Here's the drawing with two shaded views (mm, measured from the low corner). I have some questions. Coordinates: 2 decimals unless noted, no trailing zeros. Order: outer loops, then holes, each group sorted by start corner. A loop starts at its lowest first (then second) coordinate and runs counter-clockwise, first axis right, second up. Notation, with made-up numbers: (-22.75, -9.5) -> (-8.75, -9.5) arc R36 ccw to (-8.75, 29.5) -> close; hole circle Ø7 at (46.25, -32). An arc over 180 degrees is marked (long way). Answer as a JSON object with one key per item and string values. Group by question number.
(1) I want a section at A-A, the plane z = 2.1. List the corners of the cut face in (x, y) for me.
(2) I want a section at B-B, the plane y = 5.5. List the corners of the cut face in (x, z) for me, plus the area to 3 significant figures.
(3) I need wall thicknesses on line 1 (X direction, y = 2, z = 1.25); line 2 (Y direction, x = 4.3, z = 2.3); line 3 (Y direction, x = 14.5, z = 0.65). Which ranges of each line are inside material? Lowest first, please.
(4) I want a section at C-C, the plane x = 39. List the corners of the cut face in (y, z) for me.
(5) For pin 1 (2 mm diameter, centred on x = 42, y = 4.5, fed in from +Z); pin 2 (4.5 mm diameter, centred on x = 4.3, y = 4.3, fed in from +Z); pin 3 (2 mm diameter, centred on x = 34, y = 3.5, fed in from -Z); pin 4 (1 mm diameter, centred on y = 3, z = 1, fed in from -X), each with a flat end and sliding along its axis, tell me the tip position at first contact or that it passes through.
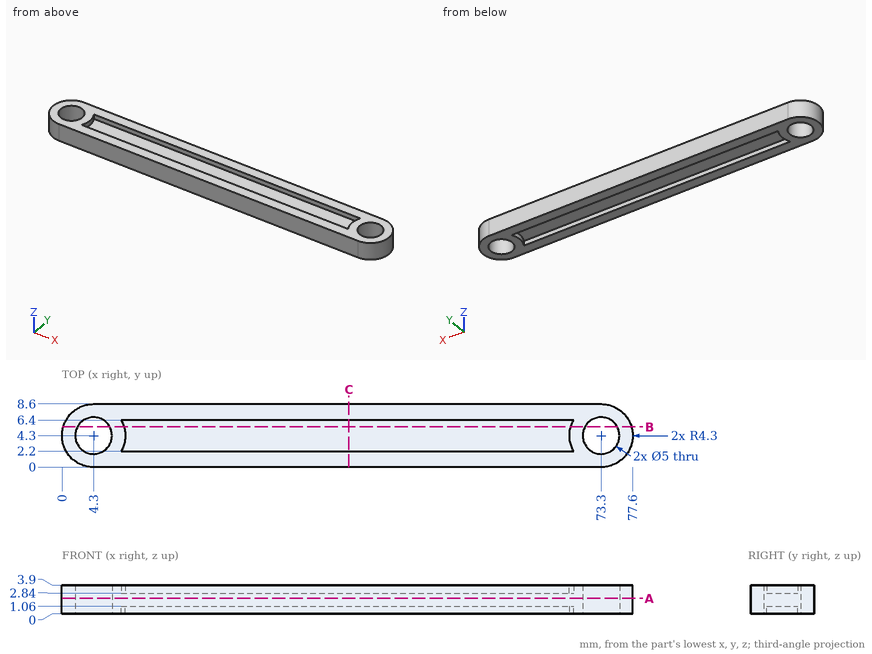
Computed values:
{
 "1": {"outline": "(4.3, 0) -> (73.3, 0) arc R4.3 ccw to (73.3, 8.6) -> (4.3, 8.6) arc R4.3 ccw to start; hole circle Ø5 at (4.3, 4.3); hole circle Ø5 at (73.3, 4.3)"},
 "2": {"outline": "(0.17, 0) -> (2.11, 0) -> (2.11, 3.9) -> (0.17, 3.9) -> close; (6.49, 0) -> (8.43, 0) -> (8.43, 1.06) -> (69.17, 1.06) -> (69.17, 0) -> (71.11, 0) -> (71.11, 3.9) -> (69.17, 3.9) -> (69.17, 2.84) -> (8.43, 2.84) -> (8.43, 3.9) -> (6.49, 3.9) -> close; (75.49, 0) -> (77.43, 0) -> (77.43, 3.9) -> (75.49, 3.9) -> close", "area": "138 mm2"},
 "3": {"line 1": "x = 0.67 to 3.32, 5.28 to 72.32, 74.28 to 76.93", "line 2": "y = 0 to 1.8, 6.8 to 8.6", "line 3": "y = 0 to 2.2, 6.4 to 8.6"},
 "4": {"outline": "(0, 0) -> (2.2, 0) -> (2.2, 1.06) -> (6.4, 1.06) -> (6.4, 0) -> (8.6, 0) -> (8.6, 3.9) -> (6.4, 3.9) -> (6.4, 2.84) -> (2.2, 2.84) -> (2.2, 3.9) -> (0, 3.9) -> close"},
 "5": {"pin 1": "stops at z = 2.84", "pin 2": "passes through", "pin 3": "stops at z = 1.06", "pin 4": "stops at x = 0.08"}
}
